Geometry: final body of the model. Coordinates: model frame, mm. A direction names the side the tool comes from. Round coordinates to 2 decimals unless told otherwise and drop trailing zeros. Write each loop counter-clockwise with the first axis right and the second up, starting at its lowest first coordinate (ties: lowest second). Pieces come first, ordered by that corner, then holes.
from build123d import *

# Parameters (mm, degrees)
SKETCH1_R           = 1.6
SKETCH1_R_2         = 1.5
BOSS_EXTRUDE1_DEPTH = 3.5
SKETCH2_R           = 7.5
CUT_EXTRUDE1_DEPTH  = 10
BOSS_EXTRUDE2_DEPTH = 6
CUT_EXTRUDE2_DEPTH  = 6


with BuildPart() as part:
    # Sketch1 → Boss-Extrude1 (new body)
    with BuildSketch(Plane.XY):
        with BuildLine():
            Line((50, -45), (-50, -45))
            ThreePointArc((-50, -45), (-53.535533906, -43.535533906), (-55, -40))
            Line((-55, -40), (-55, 40))
            ThreePointArc((-55, 40), (-53.535533906, 43.535533906), (-50, 45))
            Line((-50, 45), (50, 45))
            ThreePointArc((50, 45), (53.535533906, 43.535533906), (55, 40))
            Line((55, 40), (55, -40))
            ThreePointArc((55, -40), (53.535533906, -43.535533906), (50, -45))
        make_face()
        with Locations((-46.5, 36.5)):
            Circle(SKETCH1_R, mode=Mode.SUBTRACT)
        with Locations((46.5, 36.5)):
            Circle(SKETCH1_R, mode=Mode.SUBTRACT)
        with Locations(Location((46.5, -36.5, 0), (0, 0, 180))):
            Circle(SKETCH1_R, mode=Mode.SUBTRACT)
        with Locations(Location((-46.5, -36.5, 0), (0, 0, 180))):
            Circle(SKETCH1_R, mode=Mode.SUBTRACT)
        with Locations((38.05, 13.55)):
            Circle(SKETCH1_R_2, mode=Mode.SUBTRACT)
        with Locations((38.05, -13.55)):
            Circle(SKETCH1_R_2, mode=Mode.SUBTRACT)
        with Locations(Location((-38.05, -13.55, 0), (0, 0, 180))):
            Circle(SKETCH1_R_2, mode=Mode.SUBTRACT)
        with Locations(Location((-38.05, 13.55, 0), (0, 0, 180))):
            Circle(SKETCH1_R_2, mode=Mode.SUBTRACT)
    extrude(amount=BOSS_EXTRUDE1_DEPTH)

    # Sketch2 → Cut-Extrude1 (cut)
    with BuildSketch(Plane(origin=(0, 0, 0), x_dir=(-1, 0, 0), z_dir=(0, 0, -1))):
        with Locations((0, 30)):
            Circle(SKETCH2_R)
        with BuildLine():
            Line((-15, -15), (15, -15))
            ThreePointArc((15, -15), (18.535533906, -13.535533906), (20, -10))
            Line((20, -10), (20, 10))
            ThreePointArc((20, 10), (18.535533906, 13.535533906), (15, 15))
            Line((15, 15), (-15, 15))
            ThreePointArc((-15, 15), (-18.535533906, 13.535533906), (-20, 10))
            Line((-20, 10), (-20, -10))
            ThreePointArc((-20, -10), (-18.535533906, -13.535533906), (-15, -15))
        make_face()
        with BuildLine():
            Line((1.732050808, -39), (8.660254038, -27))
            ThreePointArc((8.660254038, -27), (8.660254038, -25), (6.92820323, -24))
            Line((6.92820323, -24), (-6.92820323, -24))
            ThreePointArc((-6.92820323, -24), (-8.660254038, -25), (-8.660254038, -27))
            Line((-8.660254038, -27), (-1.732050808, -39))
            ThreePointArc((-1.732050808, -39), (0, -40), (1.732050808, -39))
        make_face()
    extrude(amount=-CUT_EXTRUDE1_DEPTH, mode=Mode.SUBTRACT)

    # Sketch3 → Boss-Extrude2 (add)
    with BuildSketch(Plane.XY.offset(3.5)):
        with BuildLine():
            Line((50, -45), (-50, -45))
            ThreePointArc((-50, -45), (-53.535533906, -43.535533906), (-55, -40))
            Line((-55, -40), (-55, 40))
            ThreePointArc((-55, 40), (-53.535533906, 43.535533906), (-50, 45))
            Line((-50, 45), (50, 45))
            ThreePointArc((50, 45), (53.535533906, 43.535533906), (55, 40))
            Line((55, 40), (55, -40))
            ThreePointArc((55, -40), (53.535533906, -43.535533906), (50, -45))
        make_face()
    extrude(amount=BOSS_EXTRUDE2_DEPTH)

    # Sketch4 → Cut-Extrude2 (cut)
    with BuildSketch(Plane.XY.offset(9.5)):
        with BuildLine():
            Line((47.5, -42.5), (-47.5, -42.5))
            ThreePointArc((-47.5, -42.5), (-51.035533906, -41.035533906), (-52.5, -37.5))
            Line((-52.5, -37.5), (-52.5, 37.5))
            ThreePointArc((-52.5, 37.5), (-51.035533906, 41.035533906), (-47.5, 42.5))
            Line((-47.5, 42.5), (47.5, 42.5))
            ThreePointArc((47.5, 42.5), (51.035533906, 41.035533906), (52.5, 37.5))
            Line((52.5, 37.5), (52.5, -37.5))
            ThreePointArc((52.5, -37.5), (51.035533906, -41.035533906), (47.5, -42.5))
        make_face()
    extrude(amount=-CUT_EXTRUDE2_DEPTH, mode=Mode.SUBTRACT)


solid = part.part
1) Section A-A on y = -7. Output: boundary loops of the cut face in (x, z).
2) Reachability of faces 1 (the flat face through (5.245, -32.916, 1.726)), 2 (the flat face through (1, -42.5, 7)), 3 (the flat face through (1, 21, 0)) from +Z, -Z, +X, -X, +Y, -Y: full face, straight path, thin tool, end or side. Return the list, or none.
3) Section B-B on z = 1.75. State how many separate pieces and enclosed holes the cut face has, plus the area to 3 significant figures.
4) Section C-C on x = 38.05. Output: boundary loops of the cut face in (y, z), plus the area to 3 significant figures.
5) Line query: probe 1 along Y at (x, z) = (46.5, 1.2); probe 2 along Y at (x, z) = (38.05, 2.7); probe 3 along Y at (x, z) = (43, 5.75). Output: solid intervals per line, ascending.
6) First-contact query: P1, Ø5, axis at x = 46.5, y = 36.5, coming from the -Z side; P2, Ø2.5, axis at x = -38.05, y = 13.55, coming from the -Z side; P3, Ø1, axis at x = 11, y = 20.5, coming from the +Z side. Flat tips, straight axial feed; report the tip coordinate or a pass-through.
7) Section D-D on z = 7.25. Output: boundary loops of the cut face in (x, y), plus the area to 3 significant figures.
8) Draft query along Y for faces 4 (the cylindrical face through (53, 44, 5)), 5 (the flat face through (-55, -1, 5)), 6 (the cylindrical face through (51.07, -41, 6.54)). Return one class per face: pulls with the +Y half, pulls with the -Y half, needs draft (parallel to the pull), parting line crosses it, or undercut.
Filled in:
1. outline: (-55, 0) - (-20, 0) - (-20, 3.5) - (-52.5, 3.5) - (-52.5, 9.5) - (-55, 9.5) - close; (20, 0) - (55, 0) - (55, 9.5) - (52.5, 9.5) - (52.5, 3.5) - (20, 3.5) - close
2. face 1: +Z, -Z
2. face 2: +Z
2. face 3: -Z, +X, -X, +Y, -Y
3. separate pieces: 1
3. enclosed holes: 11
3. area: 8,280 mm2
4. outline: (-45, 0) - (-15.05, 0) - (-15.05, 3.5) - (-42.5, 3.5) - (-42.5, 9.5) - (-45, 9.5) - close; (-12.05, 0) - (12.05, 0) - (12.05, 3.5) - (-12.05, 3.5) - close; (15.05, 0) - (45, 0) - (45, 9.5) - (42.5, 9.5) - (42.5, 3.5) - (15.05, 3.5) - close
4. area: 324 mm2
5. probe 1: y = -45 to -38.1, -34.9 to 34.9, 38.1 to 45
5. probe 2: y = -45 to -15.05, -12.05 to 12.05, 15.05 to 45
5. probe 3: y = -45 to -42.5, 42.5 to 45
6. P1: stops at z = 0
6. P2: passes through
6. P3: stops at z = 3.5
7. outline: (-55, -40) arc R5 ccw to (-50, -45) - (50, -45) arc R5 ccw to (55, -40) - (55, 40) arc R5 ccw to (50, 45) - (-50, 45) arc R5 ccw to (-55, 40) - close; hole (-52.5, -37.5) arc R5 ccw to (-47.5, -42.5) - (47.5, -42.5) arc R5 ccw to (52.5, -37.5) - (52.5, 37.5) arc R5 ccw to (47.5, 42.5) - (-47.5, 42.5) arc R5 ccw to (-52.5, 37.5) - close
7. area: 975 mm2
8. face 4: pulls with the +Y half
8. face 5: needs draft
8. face 6: undercut
